Here's how the part is built. I have some questions about the finished solid (model axes, mm). A direction names the side the tool comes from. Coordinates: 2 decimals unless noted, no trailing zeros. Order: outer loops, then holes, each group sorted by start corner. A loop starts at its lowest first (then second) coordinate and runs counter-clockwise, first axis right, second up. Notation, with made-up numbers: (-22.75, 73) - (-10.75, 73) arc R12 ccw to (-10.75, 79) - close; hole circle Ø6 at (-18.75, 33). An arc over 180 degrees is marked (long way). Answer as CSV lines item,"result". Start each with the question number.
Q1. I need wall thicknesses on line 1 (Y direction, x = -42, z = 0.2); line 2 (Y direction, x = 27, z = 1.95); line 3 (X direction, y = 43, z = 0.75). Which ranges of each line are inside material? Lowest first, please.
Q2. Suppose I cut it at C-C (z = 0.6). Count the separate pieces of the cut face and the enclosed holes in it, then the cut area to 3 significant figures.
Q3. For pin 1 Ø4 at (x, y) = (41.77, -26.5) entering from -Z, with a flat end and sliding along its axis, tell me the tip position at first contact or that it passes through.
Q4. Suppose I cut it at D-D (y = 22.5). Please give me the cut outline in (x, z), then the cut area to 3 significant figures.
Q5. Suppose I cut it at B-B (x = -11). Please give me the cut outline in (y, z).
Q6. Thinking about a two-plate mould opening in Y: for faces 3 (the face through (-43.664, -26.049, 1.479)), 4 (the face through (40.336, -26.049, 1.479)), 5 (the face through (-1, 47.5, 1)), 6 (the face through (-1, 11, 0)), which applies, released by +Y, released by -Y, zero draft, split by the parting line, or undercut?
Q7. For faces 1 (the face through (-1, -47.5, 1)), 2 (the face through (-1, -2.55, 2)), which set-ups out of +Z, -Z, +X, -X, +Y, -Y let a thin tool reach every point of the face, with its end or its side?
Q8. Suppose I cut it at A-A (y = -26.5). Please give me the cut outline in (x, z), then the cut area to 3 significant figures.
from build123d import *

# Parameters (mm, degrees)
SKETCH_1_W          = 130
SKETCH_1_H          = 95
EXTRUDE_1_DEPTH     = 3
SKETCH_3_R          = 1.5
CUT_EXTRUDE_2_DEPTH = 10
SKETCH_4_R          = 1.5
CUT_EXTRUDE_3_DEPTH = 10
SKETCH_5_W          = 100
SKETCH_5_H          = 5.1
CUT_EXTRUDE_4_DEPTH = 10
FILLET_1_R          = 1
FILLET_2_R          = 1


with BuildPart() as part:
    # 草图1 → 凸台-拉伸1 (new body)
    with BuildSketch(Plane.XY):
        Rectangle(SKETCH_1_W, SKETCH_1_H)
    extrude(amount=EXTRUDE_1_DEPTH)

    # 草图3 → 切除-拉伸2 (cut)
    with BuildSketch(Plane(origin=(0, 0, 0), x_dir=(-1, 0, 0), z_dir=(0, 0, -1))):
        with Locations((-57.767112616, -26.5)):
            Circle(SKETCH_3_R)
        with Locations((-41.767112616, -26.5)):
            Circle(SKETCH_3_R)
        with Locations((42.232887384, -26.5)):
            Circle(SKETCH_3_R)
        with Locations((58.232887384, -26.5)):
            Circle(SKETCH_3_R)
    extrude(amount=-CUT_EXTRUDE_2_DEPTH, mode=Mode.SUBTRACT)

    # 草图4 → 切除-拉伸3 (cut)
    with BuildSketch(Plane(origin=(0, 0, 0), x_dir=(-1, 0, 0), z_dir=(0, 0, -1))):
        with Locations((-46.767112616, 42.5)):
            Circle(SKETCH_4_R)
        with Locations((-46.767112616, 22.5)):
            Circle(SKETCH_4_R)
        with Locations((47.232887384, 42.5)):
            Circle(SKETCH_4_R)
        with Locations((47.232887384, 22.5)):
            Circle(SKETCH_4_R)
    extrude(amount=-CUT_EXTRUDE_3_DEPTH, mode=Mode.SUBTRACT)

    # 草图5 → 切除-拉伸4 (cut)
    with BuildSketch(Plane.XY.offset(3)):
        Rectangle(SKETCH_5_W, SKETCH_5_H)
    extrude(amount=-CUT_EXTRUDE_4_DEPTH, mode=Mode.SUBTRACT)

    # 圆角1
    fillet_1_edges = [part.edges().sort_by_distance(p)[0] for p in [
        (-50, 2.55, 1.5),
    ]]
    fillet(fillet_1_edges, radius=FILLET_1_R)

    # 圆角2
    fillet_2_edges = [part.edges().sort_by_distance(p)[0] for p in [
        (-50, -2.55, 1.5),
        (50, 2.55, 1.5),
        (50, -2.55, 1.5),
    ]]
    fillet(fillet_2_edges, radius=FILLET_2_R)


solid = part.part
Here are the results:
1,line 1,"y = -47.5 to -27.98, -25.02 to -2.55, 2.55 to 47.5"
1,line 2,"y = -47.5 to -2.55, 2.55 to 47.5"
1,line 3,"x = -65 to -48.65, -45.82 to 45.35, 48.18 to 65"
2,separate pieces,"1"
2,enclosed holes,"9"
2,area,"11,800 mm²"
3,pin 1,"stops at z = 0"
4,outline,"(-65, 0) - (-48.73, 0) - (-48.73, 3) - (-65, 3) - close; (-45.73, 0) - (45.27, 0) - (45.27, 3) - (-45.73, 3) - close; (48.27, 0) - (65, 0) - (65, 3) - (48.27, 3) - close"
4,area,"372 mm²"
5,outline,"(-47.5, 0) - (-2.55, 0) - (-2.55, 3) - (-47.5, 3) - close; (2.55, 0) - (47.5, 0) - (47.5, 3) - (2.55, 3) - close"
6,face 3,"undercut"
6,face 4,"undercut"
6,face 5,"released by +Y"
6,face 6,"zero draft"
7,face 1,"+Z, -Z, +X, -X, -Y"
7,face 2,"+Z, -Z"
8,outline,"(-65, 0) - (-59.73, 0) - (-59.73, 3) - (-65, 3) - close; (-56.73, 0) - (-43.73, 0) - (-43.73, 3) - (-56.73, 3) - close; (-40.73, 0) - (40.27, 0) - (40.27, 3) - (-40.73, 3) - close; (43.27, 0) - (56.27, 0) - (56.27, 3) - (43.27, 3) - close; (59.27, 0) - (65, 0) - (65, 3) - (59.27, 3) - close"
8,area,"354 mm²"
